For this review, take the finished solid that the model builds, in its own axes (mm). Face numbers are marked on the shaded views. Round coordinates to 2 decimals unless told otherwise and drop trailing zeros.
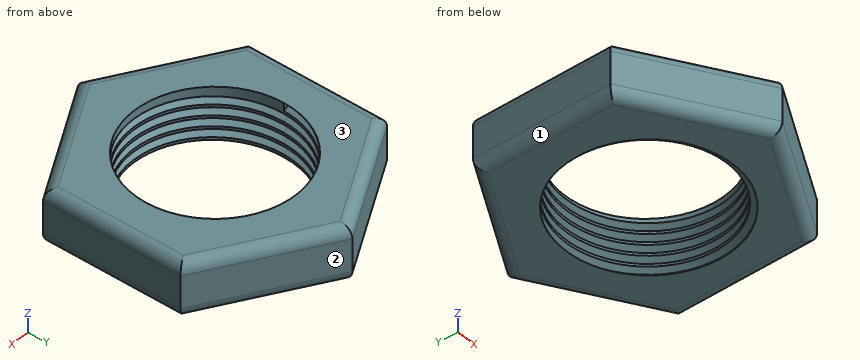
from build123d import *

# Parameters (mm, degrees)
IZIM1_R                     = 15
Y_KSEKLIK_EKSTR_ZYON1_DEPTH = 10
DI_2_PITCH                  = 2
RADYUS1_R                   = 2
RADYUS3_R                   = 2


with BuildPart() as part:
    # Çizim1 → Yükseklik-Ekstrüzyon1 (new body)
    with BuildSketch(Plane.XY):
        Polygon((0, 25.980762114), (-22.5, 12.990381057), (-22.5, -12.990381057), (0, -25.980762114), (22.5, -12.990381057), (22.5, 12.990381057), align=None)
        Circle(IZIM1_R, mode=Mode.SUBTRACT)
    extrude(amount=Y_KSEKLIK_EKSTR_ZYON1_DEPTH)

    # Diş2: the profile of Diş Profili2 profile screwed along a right-hand helix of 5 turns, 10 arcs to a turn; built about Z, then put on its axis
    di_2_z = Axis((0, 0, 0), (0, 0, 1))
    di_2_corners = [(14.9997, 0, -0.000173205), (16.08253175, 0, 0.624999997), (16.08253175, 0, 0.874999997), (14.9997, 0, 1.5001732)]
    with BuildLine(mode=Mode.PRIVATE) as di_2_profile:
        Line(di_2_corners[0], di_2_corners[1])
        Line(di_2_corners[1], di_2_corners[2])
        Line(di_2_corners[2], di_2_corners[3])
        Line(di_2_corners[3], di_2_corners[0])
    di_2_cap = Face(di_2_profile.wire())
    di_2_turn_angles = [0, 18, 36, 54, 72, 90, 108, 126, 144, 162, 180, 198, 216, 234, 252, 270, 288, 306, 324, 342, 360]
    di_2_turn_weights = [1, 0.9510565162951535, 1, 0.9510565162951535, 1, 0.9510565162951535, 1, 0.9510565162951535, 1, 0.9510565162951535, 1, 0.9510565162951535, 1, 0.9510565162951535, 1, 0.9510565162951535, 1, 0.9510565162951535, 1, 0.9510565162951535, 1]
    di_2_turn_rails = [Edge.make_bspline([Vector(p[0], p[1], 0).rotate(di_2_z, di_2_turn_angles[k]) / di_2_turn_weights[k] + Vector(0, 0, p[2] + DI_2_PITCH * di_2_turn_angles[k] / 360) for k in range(21)], [0, 0, 0, 1, 1, 2, 2, 3, 3, 4, 4, 5, 5, 6, 6, 7, 7, 8, 8, 9, 9, 10, 10, 10], 2, di_2_turn_weights) for p in di_2_corners]
    di_2_turn_sides = [Face.make_surface_from_curves(di_2_turn_rails[p[0]], di_2_turn_rails[p[1]]) for p in [(0, 1), (1, 2), (2, 3), (3, 0)]]
    di_2 = Plane(origin=(0, 0, 10), x_dir=(-1, 0, 0), z_dir=(0, 0, -1)) * Solid(Shell([*[p.moved(Location((0, 0, DI_2_PITCH * i))) for i in range(5) for p in di_2_turn_sides], di_2_cap, di_2_cap.rotate(di_2_z, 1800).moved(Location((0, 0, DI_2_PITCH * 1800 / 360)))]))
    add(di_2, mode=Mode.SUBTRACT)

    # Radyus1
    radyus1_edges = [part.edges().sort_by_distance(p)[0] for p in [
        (-22.5, 0, 10),
        (-11.25, -19.485571585, 10),
        (11.25, -19.485571585, 10),
        (22.5, 0, 10),
        (11.25, 19.485571585, 10),
        (-11.25, 19.485571585, 10),
    ]]
    fillet(radyus1_edges, radius=RADYUS1_R)

    # Radyus3
    radyus3_edges = [part.edges().sort_by_distance(p)[0] for p in [
        (22.5, 0, 0),
        (11.25, -19.485571585, 0),
        (-11.25, -19.485571585, 0),
        (-22.5, 0, 0),
        (-11.25, 19.485571585, 0),
        (11.25, 19.485571585, 0),
    ]]
    fillet(radyus3_edges, radius=RADYUS3_R)


solid = part.part
(1) Clearance check with flat-ended pins moving along their axes: P1, Ø4, axis at y = 16, z = 1.5, coming from the -X side; P2, Ø4, axis at x = -7, z = 6, coming from the +Y side; P3, Ø3, axis at x = -9.5, z = 8.5, coming from the -Y side; P4, Ø24, axis at x = 0, y = 0, coming from the +Z side. State where each tip first meets the part, or that it passes through.
(2) Wall thickness on L1, parallel to Z at x = 17, y = 14; L2, parallel to X at y = 0, z = 3.7; L3, parallel to X at y = 5, z = 4: over which ranges is each line inside the solid? List them lowest first.
(3) Draft analysis for pull direction Z (two halves, no side actions). For the marked faces 1, 2 and 3, state which applies: pulls with the +Z half, pulls with the -Z half, needs draft (parallel to the pull), parting line crosses it, or undercut.
Here are the results:
1. P1: stops at x = -20.69
1. P2: stops at y = 23.09
1. P3: stops at y = -21.33
1. P4: passes through
2. L1: z = 0 to 10
2. L2: x = -22.5 to -15.52, 15.35 to 22.5
2. L3: x = -22.5 to -14.14, 14.87 to 22.5
3. face 1: pulls with the -Z half
3. face 2: needs draft
3. face 3: pulls with the +Z half
